```python
from build123d import *

# Parameters (mm, degrees)
BOSS_EXTRU_1_DEPTH      = 3.81
ESQUISSE2_R             = 7.62
BOSS_EXTRU_2_DEPTH      = 1.27
ESQUISSE3_R             = 4.826
BOSS_EXTRU_3_DEPTH      = 1.27
ESQUISSE4_R             = 5.334
BOSS_EXTRU_4_DEPTH      = 1.27
ESQUISSE5_R             = 2
ENL_V_MAT_EXTRU_1_DEPTH = 12.43


with BuildPart() as part:
    # Esquisse1 → Boss.-Extru.1 (new body, symmetric)
    with BuildSketch(Plane.XY):
        Polygon((7.332348419, 0), (3.666174209, 6.35), (-3.666174209, 6.35), (-7.332348419, 0), (-3.666174209, -6.35), (3.666174209, -6.35), align=None)
    extrude(amount=BOSS_EXTRU_1_DEPTH, both=True)

    # Esquisse2 → Boss.-Extru.2 (add)
    with BuildSketch(Plane(origin=(0, 0, -3.81), x_dir=(-1, 0, 0), z_dir=(0, 0, -1))):
        Circle(ESQUISSE2_R)
    extrude(amount=BOSS_EXTRU_2_DEPTH)

    # Esquisse3 → Boss.-Extru.3 (add)
    with BuildSketch(Plane.XY.offset(3.81)):
        Circle(ESQUISSE3_R)
    extrude(amount=BOSS_EXTRU_3_DEPTH)

    # Esquisse4 → Boss.-Extru.4 (add)
    with BuildSketch(Plane.XY.offset(5.08)):
        Circle(ESQUISSE4_R)
    extrude(amount=BOSS_EXTRU_4_DEPTH)

    # Esquisse5 → Enlèv. mat.-Extru.1 (cut, through all)
    with BuildSketch(Plane(origin=(0, 0, -5.08), x_dir=(-1, 0, 0), z_dir=(0, 0, -1))):
        Circle(ESQUISSE5_R)
    extrude(amount=-ENL_V_MAT_EXTRU_1_DEPTH, mode=Mode.SUBTRACT)


solid = part.part
```
Could you check a few things on this model? Use its own coordinates, in mm. A direction names the side the tool comes from. Coordinates: 2 decimals unless noted, no trailing zeros. Loops run counter-clockwise (first coordinate to the right, second up) from the corner with the lowest first, then second, coordinate; pieces in that order, holes last. Notation, with made-up numbers: M 87.5,65 L 127.5,65 A23 ccw 127.5,102 Z; hole C 77,-28 d2. An arc over 180 degrees is marked long. Put each result on its own line as item: value. Start each with the question number.
(1) Suppose I cut it at C-C on z = -0.5. Please give me the cut outline in (x, y).
(2) I need wall thicknesses on line 1 (Y direction, x = 0, z = -0.75); line 2 (Z direction, x = 5.5, y = -1.5); line 3 (Z direction, x = 0, y = -5). Which ranges of each line are inside material? Lowest first, please. Write a range as from..to.
(3) Thinking about a two-plate mould opening in Z: for faces 1 (the face through (-3.83, -2.937, 4.436)), 2 (the face through (2.3, 0.1, 6.35)), 3 (the face through (5, 1, 3.81)), 4 (the face through (5.474, -3.219, 0.053)), which applies, pulls with the +Z half, pulls with the -Z half, needs draft (parallel to the pull), parting line crosses it, or undercut?
(4) Will these pins go through, and if not, where does the flat tip stop? P1, Ø1.5, axis at y = -2.5, z = -2, coming from the -X side; P2, Ø1.5, axis at y = -2.5, z = 1, coming from the +X side; P3, Ø1.5, axis at y = 4.5, z = -3.5, coming from the -X side (3 decimals); P4, Ø2.5, axis at x = 0, y = 0, coming from the +Z side (3 decimals).
(5) Suppose I cut it at B-B on y = 0.25. Please give me the cut outline in (x, z), then the cut area to 3 significant figures.
(6) Suppose I cut it at D-D on y = 6. Please give me the cut outline in (x, z), then the cut area to 3 significant figures.
(7) Suppose I cut it at A-A on x = 0. Please give me the cut outline in (y, z).
(8) For faces 5 (the face through (-5.525, -3.131, 0.053)), 6 (the face through (-4, -3, 5.08)), 7 (the face through (-6, -3, -3.81)), 8 (the face through (0, -6.35, 0)), which set-ups out of +Z, -Z, +X, -X, +Y, -Y let a thin tool reach every point of the face, with its end or its side?
Solutions:
1. outline: M -7.33,0 L -3.67,-6.35 L 3.67,-6.35 L 7.33,0 L 3.67,6.35 L -3.67,6.35 Z; hole C 0,0 d4
2. line 1: y = -6.35..-2, 2..6.35
2. line 2: z = -5.08..3.81
2. line 3: z = -5.08..3.81, 5.08..6.35
3. face 1: undercut
3. face 2: pulls with the +Z half
3. face 3: undercut
3. face 4: needs draft
4. P1: stops at x = -6.32
4. P2: stops at x = 6.32
4. P3: stops at x = -6.595
4. P4: passes through
5. outline: M -7.62,-5.08 L -1.98,-5.08 L -1.98,6.35 L -5.33,6.35 L -5.33,5.08 L -4.82,5.08 L -4.82,3.81 L -7.19,3.81 L -7.19,-3.81 L -7.62,-3.81 Z; M 1.98,-5.08 L 7.62,-5.08 L 7.62,-3.81 L 7.19,-3.81 L 7.19,3.81 L 4.82,3.81 L 4.82,5.08 L 5.33,5.08 L 5.33,6.35 L 1.98,6.35 Z
5. area: 109 mm2
6. outline: M -4.7,-5.08 L 4.7,-5.08 L 4.7,-3.81 L 3.87,-3.81 L 3.87,3.81 L -3.87,3.81 L -3.87,-3.81 L -4.7,-3.81 Z
6. area: 70.9 mm2
7. outline: M -7.62,-5.08 L -2,-5.08 L -2,6.35 L -5.33,6.35 L -5.33,5.08 L -4.83,5.08 L -4.83,3.81 L -6.35,3.81 L -6.35,-3.81 L -7.62,-3.81 Z; M 2,-5.08 L 7.62,-5.08 L 7.62,-3.81 L 6.35,-3.81 L 6.35,3.81 L 4.83,3.81 L 4.83,5.08 L 5.33,5.08 L 5.33,6.35 L 2,6.35 Z
8. face 5: +Z, -X, -Y
8. face 6: none
8. face 7: +Z
8. face 8: +Z, +X, -X, -Y
